Could you check a few things on this model? Use its own coordinates, in mm. Face numbers are marked on the shaded views. A direction names the side the tool comes from. Coordinates: 2 decimals unless noted, no trailing zeros. Write each loop counter-clockwise with the first axis right and the second up, starting at its lowest first coordinate (ties: lowest second). Pieces come first, ordered by that corner, then holes.
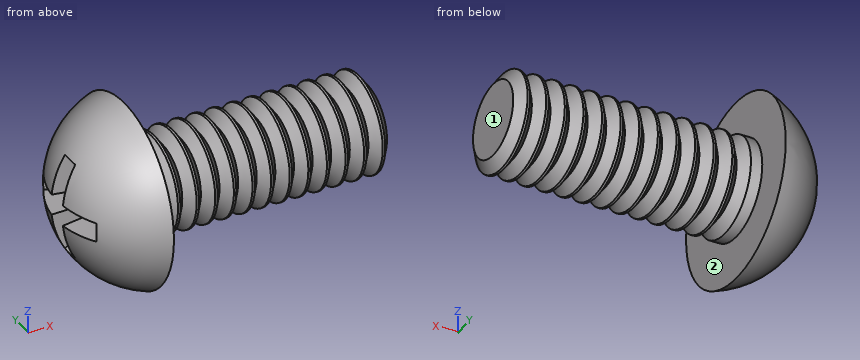
```python
from build123d import *

# Parameters (mm, degrees)
CIRPATTERN1_COUNT = 2
CIRPATTERN1_ANGLE = 90
THDSCHPAT_COUNT   = 13
THDSCHPAT_PITCH   = 1.217083333


with BuildPart() as part:
    # BodySke → Base-Revolve (revolve)
    with BuildSketch(Plane.XY):
        with BuildLine():
            Line((20.32, 0), (20.32, 3.175))
            Line((20.32, 3.175), (4.445, 3.175))
            Line((4.445, 3.175), (4.445, 5.9944))
            ThreePointArc((4.445, 5.9944), (1.232493041, 3.73131533), (0, 0))
            Line((0, 0), (20.32, 0))
        make_face()
    revolve(axis=Axis((0, 0, 0), (1, 0, 0)))

    # Sketch3 → Cross section 0
    with BuildSketch(Plane(origin=(0, 0, 0), x_dir=(0, 0, -1), z_dir=(1, 0, 0))):
        with BuildLine():
            Line((0.6858, -3.8989), (-0.6858, -3.8989))
            Line((-0.6858, -3.8989), (-0.6858, 3.8989))
            Line((-0.6858, 3.8989), (0.6858, 3.8989))
            Line((0.6858, 3.8989), (0.6858, -3.8989))
        make_face()
    # Sketch4 → Cross section 1
    with BuildSketch(Plane(origin=(4.5974, 0, 0), x_dir=(0, 0, -1), z_dir=(1, 0, 0))):
        with BuildLine():
            Line((0.3429, -0.3429), (-0.3429, -0.3429))
            Line((-0.3429, -0.3429), (-0.3429, 0.3429))
            Line((-0.3429, 0.3429), (0.3429, 0.3429))
            Line((0.3429, 0.3429), (0.3429, -0.3429))
        make_face()
    cross = loft(mode=Mode.SUBTRACT)

    # CirPattern1: Cross ×2 about axis
    cirpattern1_axis = Axis((0, 0, 0), (1, 0, 0))
    for i in range(1, CIRPATTERN1_COUNT):
        add(cross.rotate(cirpattern1_axis, i * CIRPATTERN1_ANGLE / (CIRPATTERN1_COUNT - 1)), mode=Mode.SUBTRACT)

    # ThdSchSke → ThreadSchematic (revolve, cut)
    with BuildSketch(Plane.XY, mode=Mode.PRIVATE) as threadschematic_sk:
        Polygon((5.715, -2.41935), (5.185888174, -3.175), (5.185888174, -3.96875), (6.244111826, -3.96875), (6.244111826, -3.175), align=None)
    threadschematic = revolve(threadschematic_sk.sketch.rotate(Axis((-3.175, 0, 0), (1, 0, 0)), 270), axis=Axis((-3.175, 0, 0), (1, 0, 0)), mode=Mode.SUBTRACT)

    # ThdSchPat: ThreadSchematic ×13
    with Locations(*[(i * THDSCHPAT_PITCH, 0, 0) for i in range(1, THDSCHPAT_COUNT)]):
        add(threadschematic, mode=Mode.SUBTRACT)


solid = part.part
```
1. On a 3-axis mill with a long thin cutter (end or side, diameter ignored), from which of +Z, -Z, +X, -X, +Y, -Y can I reach the whole of each face in a straight line? I mean the marked faces 1 and 2. Say none if no direction works.
Verdict:
face 1: +Z, -Z, +X, +Y, -Y
face 2: +X
2. Please list where these lines run through material, in increasing order: line 1 along Z through (x, y) = (4, 0.75); line 2 along Z through (x, y) = (1.75, -0.5); line 3 along X through (y, z) = (2.5, -2.25) (3 decimals).
Verdict:
line 1: z = -5.79 to -0.39, 0.39 to 5.79
line 2: z = -4.31 to -2.55, 2.55 to 4.31
line 3: x = 0.979 to 4.445
3. I want a section at B-B on z = -3.5. Please give me the cut outline in (x, y) (1 decimal), plus the area to 3 significant figures.
Verdict:
outline: (4.4, -4.9) - (4.4, 4.9) arc R5.2 ccw to start
area: 23.9 mm2
4. For pin 1 (1.5 mm diameter, centred on x = 16, y = -4.5, fed in from -Z); pin 2 (4 mm diameter, centred on x = 16, z = 4, fed in from +Y); pin 3 (6 mm diameter, centred on x = 5.5, z = 3, fed in from +Y); pin 4 (3 mm diameter, centred on y = 3, z = -3, fed in from +X), each with a flat end and sliding along its axis, tell me the tip position at first contact or that it passes through.
Verdict:
pin 1: passes through
pin 2: stops at y = 2.47
pin 3: stops at y = 5.99
pin 4: stops at x = 20.09
5. I want a section at A-A on y = 2.75. Give the number of separate pieces and of enclosed holes in the cut face, plus the area to 3 significant figures.
Verdict:
separate pieces: 13
enclosed holes: 0
area: 52.5 mm2
